Can you work these out from the model? Positions are in its coordinate system, mm. Face numbers are marked on the shaded views. A direction names the side the tool comes from. Round coordinates to 2 decimals unless told otherwise and drop trailing zeros. Write each loop counter-clockwise with the first axis right and the second up, starting at its lowest first coordinate (ties: lowest second). Pieces come first, ordered by that corner, then holes.
Q1. Please list where these lines run through material, in increasing order: line 1 along X through (y, z) = (2.5, -0.75); line 2 along Z through (x, y) = (-1.25, 8.7).
Q2. I'm going to push flat-ended pins straight in: pin 1 Ø0.9 at (y, z) = (3.5, -0.5) entering from +X; pin 2 Ø2 at (x, y) = (1, 9.5) entering from +Z; pin 3 Ø2 at (x, y) = (1, 9) entering from -Z. Where does each tip first touch, or does it pass through?
Q3. If we section it at C-C (y = 2.25): Please give me the cut outline in (x, z).
Q4. If we section it at D-D (x = -1.25): Please give me the cut outline in (y, z).
Q5. If we section it at A-A (x = 1.25): Please give me the cut outline in (y, z), plus the area to 3 significant figures.
Q6. For the marked faces 1, 2 and 3, which set-ups out of +Z, -Z, +X, -X, +Y, -Y let a thin tool reach every point of the face, with its end or its side?
Q7. If we section it at B-B (z = 0): Please give me the cut outline in (x, y).
Q8. We'd pull the mould along X, two halves only. Please class the marked faces 4, 5 and 6: +X half, -X half, draft (parallel to the pull), parting line (faces both ways), or undercut.
from build123d import *

# Parameters (mm, degrees)
SKETCH1_W                     = 7.5
SKETCH1_H                     = 7.5
BOSS_EXTRUDE1_DEPTH           = 7
SKETCH2_W                     = 11.5
SKETCH2_H                     = 11.5
BOSS_EXTRUDE2_DEPTH           = 3.8
SKETCH3_W                     = 6
SKETCH3_H                     = 6
CUT_EXTRUDE1_DEPTH            = 11.8
SKETCH6_W                     = 10.5
SKETCH6_H                     = 10.5
CUT_EXTRUDE3_DEPTH            = 2.8
FILLET1_R                     = 0.5
BOSS_EXTRUDE3_REACH           = 12.8
FILLET4_R                     = 1.5
FILLET2_R                     = 1
TAP_DRILL_FOR_0_80_TAP1_D     = 1.19126
TAP_DRILL_FOR_0_80_TAP1_DEPTH = 7.11
TAP_DRILL_FOR_0_80_TAP1_TIP   = 0.357890611
FILLET5_R                     = 2.25
SKETCH16_W                    = 2.5
SKETCH16_H                    = 2
CUT_EXTRUDE4_DEPTH            = 0.835786
FILLET6_R                     = 1
SKETCH17_W                    = 2
SKETCH17_H                    = 2.25
SKETCH17_H_2                  = 2.75
BOSS_EXTRUDE4_DEPTH           = 3.8
SKETCH18_R                    = 0.375
CUT_EXTRUDE5_DEPTH            = 11.8000001


with BuildPart() as part:
    # Sketch1 → Boss-Extrude1 (new body)
    with BuildSketch(Plane(origin=(0, 0, 0), x_dir=(1, 0, 0), z_dir=(0, 1, 0))):
        Rectangle(SKETCH1_W, SKETCH1_H)
    extrude(amount=BOSS_EXTRUDE1_DEPTH)

    # Sketch2 → Boss-Extrude2 (add)
    with BuildSketch(Plane(origin=(0, 7, 0), x_dir=(1, 0, 0), z_dir=(0, 1, 0))):
        Rectangle(SKETCH2_W, SKETCH2_H)
    extrude(amount=BOSS_EXTRUDE2_DEPTH)

    # Sketch3 → Cut-Extrude1 (cut, through all)
    with BuildSketch(Plane.XZ):
        Rectangle(SKETCH3_W, SKETCH3_H)
    extrude(amount=-CUT_EXTRUDE1_DEPTH, mode=Mode.SUBTRACT)

    # Sketch6 → Cut-Extrude3 (cut)
    with BuildSketch(Plane(origin=(0, 10.8, 0), x_dir=(1, 0, 0), z_dir=(0, 1, 0))):
        Rectangle(SKETCH6_W, SKETCH6_H)
    extrude(amount=-CUT_EXTRUDE3_DEPTH, mode=Mode.SUBTRACT)

    # Fillet1
    fillet1_edges = [part.edges().sort_by_distance(p)[0] for p in [
        (5.25, 9.4, 5.25),
        (5.25, 9.4, -5.25),
        (-5.25, 9.4, -5.25),
        (-5.25, 9.4, 5.25),
    ]]
    fillet(fillet1_edges, radius=FILLET1_R)

    # Sketch12 → Boss-Extrude3 (add, up to next)
    with BuildSketch(Plane.XZ, mode=Mode.PRIVATE) as boss_extrude3_sk1:
        Polygon((3.75, -3.75), (4.633883476, -2.866116524), (3.75, -1.982233047), align=None)
    boss_extrude3_tool1 = extrude(boss_extrude3_sk1.sketch, amount=-BOSS_EXTRUDE3_REACH, mode=Mode.PRIVATE) - part.part
    add(boss_extrude3_tool1.solids().sort_by_distance((4.044628, 0, -2.866117))[0])
    # Sketch12 → Boss-Extrude3 (add, up to next)
    with BuildSketch(Plane.XZ, mode=Mode.PRIVATE) as boss_extrude3_sk2:
        Polygon((2.866116524, -4.633883476), (3.75, -3.75), (1.982233047, -3.75), align=None)
    boss_extrude3_tool2 = extrude(boss_extrude3_sk2.sketch, amount=-BOSS_EXTRUDE3_REACH, mode=Mode.PRIVATE) - part.part
    add(boss_extrude3_tool2.solids().sort_by_distance((2.866117, 0, -4.044628))[0])

    # Fillet4
    fillet4_edges = [part.edges().sort_by_distance(p)[0] for p in [
        (-3, 4, 3),
        (3, 4, 3),
        (-3, 4, -3),
        (3, 4, -3),
    ]]
    fillet(fillet4_edges, radius=FILLET4_R)

    # Fillet2
    fillet2_edges = [part.edges().sort_by_distance(p)[0] for p in [
        (3.75, 3.5, -1.982233047),
        (1.982233047, 3.5, -3.75),
    ]]
    fillet(fillet2_edges, radius=FILLET2_R)

    # Tap Drill for #0-80 Tap1
    with Locations(Plane(origin=(3.75, 0, -3.75), x_dir=(-0.707106781, 0, -0.707106781), z_dir=(0.707106781, 0, -0.707106781))):
        with Locations((0, 1.25), (0, 3.75)):
            Hole(TAP_DRILL_FOR_0_80_TAP1_D / 2, depth=TAP_DRILL_FOR_0_80_TAP1_DEPTH)
            with Locations((0, 0, -(TAP_DRILL_FOR_0_80_TAP1_DEPTH + TAP_DRILL_FOR_0_80_TAP1_TIP / 2))):  # 118° drill point
                Cone(0, TAP_DRILL_FOR_0_80_TAP1_D / 2, TAP_DRILL_FOR_0_80_TAP1_TIP, mode=Mode.SUBTRACT)

    # Fillet5
    fillet5_edges = [part.edges().sort_by_distance(p)[0] for p in [
        (3.75, 3.5, 3.75),
        (-3.75, 3.5, 3.75),
        (-3.75, 3.5, -3.75),
    ]]
    fillet(fillet5_edges, radius=FILLET5_R)

    # Sketch16 → Cut-Extrude4 (cut)
    with BuildSketch(Plane(origin=(3.75, 0, -3.75), x_dir=(-0.707106781, 0, -0.707106781), z_dir=(0.707106781, 0, -0.707106781))):
        with Locations((0, 6)):
            Rectangle(SKETCH16_W, SKETCH16_H)
    extrude(amount=-CUT_EXTRUDE4_DEPTH, mode=Mode.SUBTRACT)

    # Fillet6
    fillet6_edges = [part.edges().sort_by_distance(p)[0] for p in [
        (-5.75, 8.9, -5.75),
        (-5.75, 8.9, 5.75),
        (5.75, 8.9, 5.75),
        (5.75, 8.9, -5.75),
    ]]
    fillet(fillet6_edges, radius=FILLET6_R)

    # Sketch17 → Boss-Extrude4 (add)
    with BuildSketch(Plane(origin=(0, 10.8, 0), x_dir=(1, 0, 0), z_dir=(0, 1, 0))):
        with Locations((-1.25, 6.875)):
            Rectangle(SKETCH17_W, SKETCH17_H)
        with Locations((4.75, -6.625)):
            Rectangle(SKETCH17_W, SKETCH17_H_2)
    extrude(amount=-BOSS_EXTRUDE4_DEPTH)

    # Sketch18 → Cut-Extrude5 (cut, through all)
    with BuildSketch(Plane(origin=(0, 10.8, 0), x_dir=(1, 0, 0), z_dir=(0, 1, 0))):
        with Locations((4.75, -6.375)):
            Circle(SKETCH18_R)
        with Locations((-1.25, 6.625)):
            Circle(SKETCH18_R)
    extrude(amount=-CUT_EXTRUDE5_DEPTH, mode=Mode.SUBTRACT)


solid = part.part
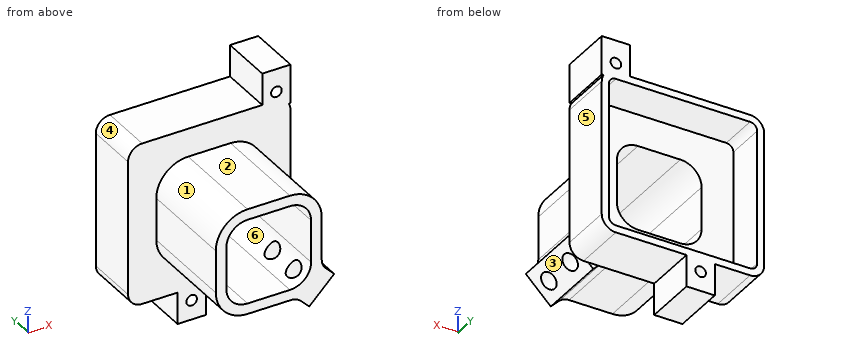
A:
1. line 1: x = -3.75 to -3, 3 to 3.75
1. line 2: z = -8 to -7, -6.25 to -5.25, 5.25 to 5.75
2. pin 1: stops at x = 3.75
2. pin 2: stops at z = 5.75
2. pin 3: stops at z = -5.75
3. outline: (-3.75, -1.5) arc R2.25 ccw to (-1.5, -3.75) - (1.57, -3.75) arc R1 cw to (2.28, -4.04) - (2.87, -4.63) - (4.63, -2.87) - (4.04, -2.28) arc R1 cw to (3.75, -1.57) - (3.75, 1.5) arc R2.25 ccw to (1.5, 3.75) - (-1.5, 3.75) arc R2.25 ccw to (-3.75, 1.5) - close; hole (-3, -1.5) arc R1.5 ccw to (-1.5, -3) - (1.5, -3) arc R1.5 ccw to (3, -1.5) - (3, 1.5) arc R1.5 ccw to (1.5, 3) - (-1.5, 3) arc R1.5 ccw to (-3, 1.5) - close
4. outline: (0, -3.75) - (7, -3.75) - (7, -6.25) - (10.8, -6.25) - (10.8, -5.25) - (8, -5.25) - (8, -3) - (0, -3) - close; (0, 3) - (8, 3) - (8, 5.25) - (10.8, 5.25) - (10.8, 5.75) - (7, 5.75) - (7, 3.75) - (0, 3.75) - close; (7, -8) - (10.8, -8) - (10.8, -7) - (7, -7) - close
5. outline: (0, -3.75) - (7, -3.75) - (7, -5.75) - (10.8, -5.75) - (10.8, -5.25) - (8, -5.25) - (8, -3) - (0, -3) - close; (0, 3) - (8, 3) - (8, 5.25) - (10.8, 5.25) - (10.8, 5.75) - (7, 5.75) - (7, 3.75) - (0, 3.75) - close
5. area: 18.8 mm2
6. face 1: +Z, -X, -Y
6. face 2: +Z, +X, -X, -Y
6. face 3: -Z, +X, -Y
7. outline: (-5.75, 7) - (-3.75, 7) - (-3.75, 0) - (-3, 0) - (-3, 8) - (-5.25, 8) - (-5.25, 10.8) - (-5.75, 10.8) - close; (3, 0) - (3.75, 0) - (3.75, 7) - (5.75, 7) - (5.75, 10.8) - (5.25, 10.8) - (5.25, 8) - (3, 8) - close
8. face 4: -X half
8. face 5: +X half
8. face 6: undercut
